Check sheet for the drawn part. Datum: minimum x, y, z corner. Units: mm. A direction names the side the tool comes from. Coordinates: 2 decimals unless noted, no trailing zeros. Write each loop counter-clockwise with the first axis right and the second up, starting at its lowest first coordinate (ties: lowest second). Pieces come first, ordered by that corner, then holes. Notation, with made-up numbers: (-25, -6.75) - (0, -6.75) arc R18 ccw to (0, 12.25) - close; hole circle Ø9 at (-26, 54). An arc over 180 degrees is marked (long way). Use one line per item in the form item = value. Start each with the question number.
1. Cross-section at A-A on y = 10. Record the boundary of the cut face in (x, z).
2. Cross-section at C-C on z = 9.5. Record the boundary of the cut face in (x, y).
3. Tool access check on the marked faces 1 and 2. Record the directions out of +Z, -Z, +X, -X, +Y, -Y that give a thin tool (end or side, any length) a straight path to the whole face; none if there is none.
4. Scan lines: line 1 along Y through (x, z) = (5.65, 37.15); line 2 along Y through (x, z) = (21, 35); line 3 along Y through (x, z) = (36, 36). Record each from-to range of solid material in increasing order.
5. Cross-section at D-D on x = 21.15. Record the boundary of the cut face in (y, z).
6. Go/stop test with flat-tipped pins: pin 1 Ø3.5 at (y, z) = (10, 9.5) entering from -X; pin 2 Ø5 at (x, y) = (36.65, 56.65) entering from -Z; pin 3 Ø2 at (x, z) = (13.5, 36) entering from -Y. Record where each tip stops, or that it passes through.
7. Cross-section at B-B on x = 5.65. Record the boundary of the cut face in (y, z), then the cut area to 3 significant figures.
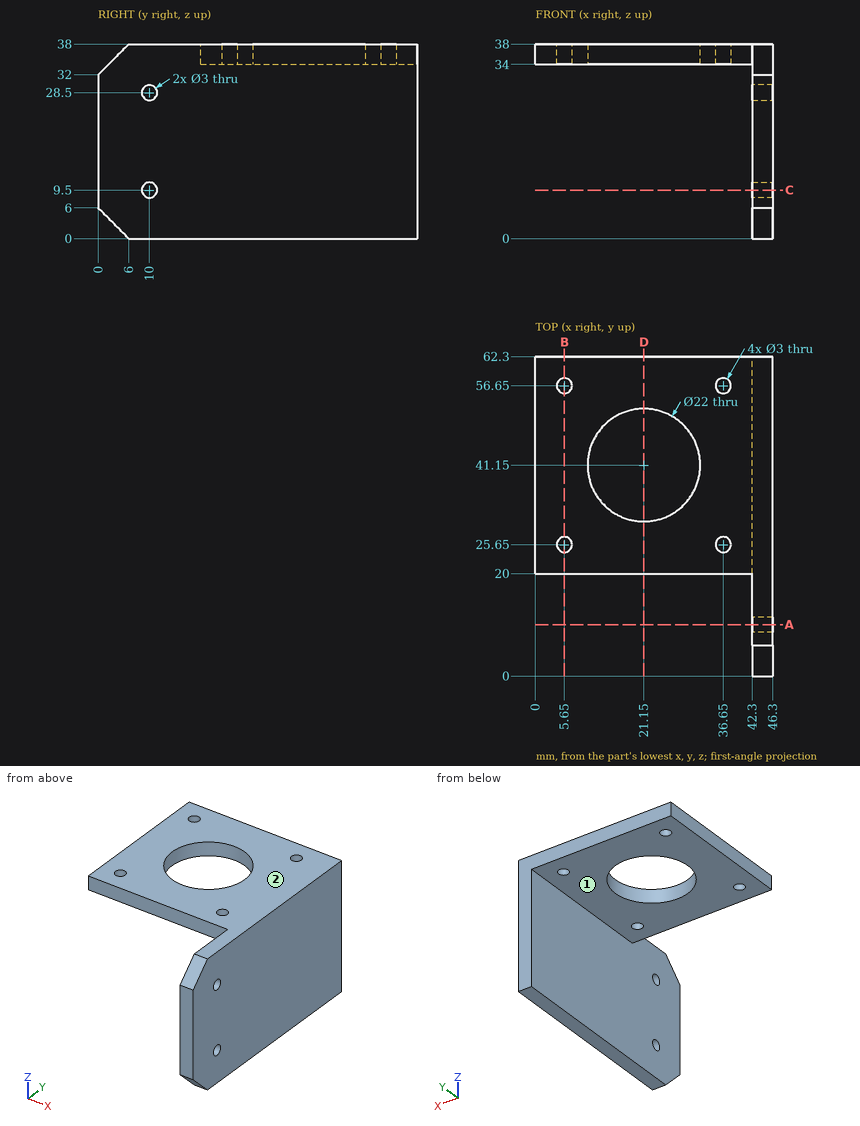
Final values:
q1.outline = (42.3, 0) - (46.3, 0) - (46.3, 8) - (42.3, 8) - close; (42.3, 11) - (46.3, 11) - (46.3, 27) - (42.3, 27) - close; (42.3, 30) - (46.3, 30) - (46.3, 38) - (42.3, 38) - close
q2.outline = (42.3, 0) - (46.3, 0) - (46.3, 8.5) - (42.3, 8.5) - close; (42.3, 11.5) - (46.3, 11.5) - (46.3, 62.3) - (42.3, 62.3) - close
q3.face_1 = -Z, -X, +Y, -Y
q3.face_2 = +Z, +X, -X, +Y, -Y
q4.line_1 = 20 to 24.15, 27.15 to 55.15, 58.15 to 62.3
q4.line_2 = 20 to 30.15, 52.15 to 62.3
q4.line_3 = 20 to 24.3, 27 to 55.3, 58 to 62.3
q5.outline = (20, 34) - (30.15, 34) - (30.15, 38) - (20, 38) - close; (52.15, 34) - (62.3, 34) - (62.3, 38) - (52.15, 38) - close
q6.pin_1 = 42.3
q6.pin_2 = 34
q6.pin_3 = 20
q7.outline = (20, 34) - (24.15, 34) - (24.15, 38) - (20, 38) - close; (27.15, 34) - (55.15, 34) - (55.15, 38) - (27.15, 38) - close; (58.15, 34) - (62.3, 34) - (62.3, 38) - (58.15, 38) - close
q7.area = 145 mm²
